Design review of the part built by this model. Coordinates are the model's own, in mm. Face numbers are marked on the shaded views. A direction names the side the tool comes from. Coordinates: 2 decimals unless noted, no trailing zeros. Loops run counter-clockwise (first coordinate to the right, second up) from the corner with the lowest first, then second, coordinate; pieces in that order, holes last. Notation, with made-up numbers: (56.25, 13.25) -> (75.25, 13.25) arc R17 ccw to (75.25, 44.25) -> close; hole circle Ø2 at (-26.75, 20). An arc over 180 degrees is marked (long way). Use one line per item in the form item = value. Start each with the question number.
1. Machinability: for the marked faces 1 and 2, which of the approach directions +Z, -Z, +X, -X, +Y, -Y give a long, thin tool a straight path to every point of the face, cutting with its end or side? Answer none if there is none.
2. Wall thickness on line 1 (Y direction, x = 60, z = 0); line 2 (X direction, y = -7.75, z = -2.75); line 3 (Y direction, x = 20, z = 4): over which ranges is each line inside the solid? List them lowest first. Write a range as from..to.
3. For pin 1 (1.5 mm diameter, centred on y = 1.5, z = 6.5, fed in from +X); pin 2 (12 mm diameter, centred on x = 63, z = 8.5, fed in from -Y); pin 3 (6 mm diameter, centred on x = 46, z = -4, fed in from -Y); pin 4 (0.7 mm diameter, centred on x = 0.5, z = -1.5, fed in from +Y), all flat-tipped, find the tip position at first contact; note any pin that passes through.
4. Consider section A-A (y = 0). State the section outline as (x, z) points, then the cut area to 3 significant figures.
5. Consider section C-C (x = 79). State the section outline as (y, z) points, then the cut area to 3 significant figures.
6. Consider section B-B (z = 0). State the section outline as (x, y) points.
from build123d import *

# Parameters (mm, degrees)
SKETCH6_W  = 24.638
SKETCH6_H  = 1.778
SLOT_DEPTH = 1.4478


with BuildPart() as part:
    # BodySke → Base-Revolve (revolve)
    with BuildSketch(Plane.XY, mode=Mode.PRIVATE) as base_revolve_sk:
        Polygon((0, 0), (0, 12.319), (0.245450977, 12.319), (7.112, 6.35), (101.6, 6.35), (101.6, 0), align=None)
    revolve(base_revolve_sk.sketch.rotate(Axis((-6.35, 0, 0), (1, 0, 0)), 90), axis=Axis((-6.35, 0, 0), (1, 0, 0)))

    # Sketch6 → Slot (cut)
    with BuildSketch(Plane.ZY):
        Rectangle(SKETCH6_W, SKETCH6_H)
    extrude(amount=-SLOT_DEPTH, mode=Mode.SUBTRACT)


solid = part.part
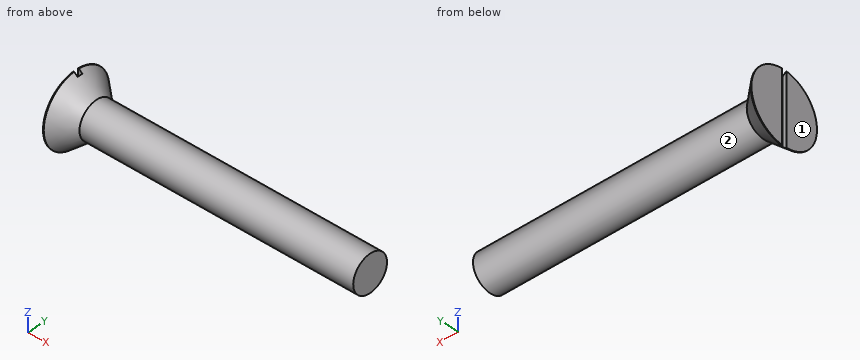
Geometry check:
q1.face_1 = +Z, -Z, -X, +Y, -Y
q1.face_2 = +X
q2.line_1 = -6.35..6.35
q2.line_2 = 0..4.96
q2.line_3 = -4.93..4.93
q3.pin_1 = 101.6
q3.pin_2 = -5.84
q3.pin_3 = -6.27
q3.pin_4 = 12.25
q4.outline = (1.45, -11.27) -> (7.11, -6.35) -> (101.6, -6.35) -> (101.6, 6.35) -> (7.11, 6.35) -> (1.45, 11.27) -> close
q4.area = 1,300 mm²
q5.outline = circle Ø12.7 at (0, 0)
q5.area = 127 mm²
q6.outline = (0, -12.32) -> (0.25, -12.32) -> (7.11, -6.35) -> (101.6, -6.35) -> (101.6, 6.35) -> (7.11, 6.35) -> (0.25, 12.32) -> (0, 12.32) -> (0, 0.89) -> (1.45, 0.89) -> (1.45, -0.89) -> (0, -0.89) -> close
